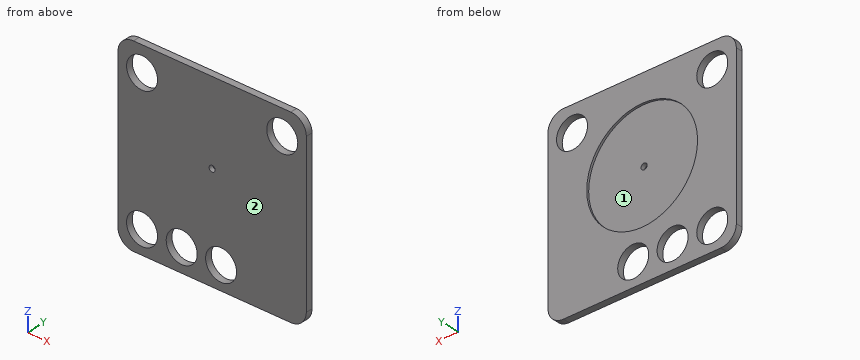
from build123d import *

# Parameters (mm, degrees)
SKETCH1_R           = 25
SKETCH1_R_2         = 7
BOSS_EXTRUDE1_DEPTH = 3
BOSS_EXTRUDE3_START = -2
SKETCH3_R           = 25
BOSS_EXTRUDE3_DEPTH = 2
SKETCH4_R           = 1.375
CUT_EXTRUDE1_DEPTH  = 2


with BuildPart() as part:
    # Sketch1 → Boss-Extrude1 (new body)
    with BuildSketch(Plane(origin=(0, 0, 0), x_dir=(1, 0, 0), z_dir=(0, 1, 0))):
        with BuildLine():
            Line((-32.846869633, -22.461451991), (38.153130367, -22.461451991))
            ThreePointArc((38.153130367, -22.461451991), (43.102877835, -20.411199459), (45.153130367, -15.461451991))
            Line((45.153130367, -15.461451991), (45.153130367, 55.538548009))
            ThreePointArc((45.153130367, 55.538548009), (43.102877835, 60.488295478), (38.153130367, 62.538548009))
            Line((38.153130367, 62.538548009), (-32.846869633, 62.538548009))
            ThreePointArc((-32.846869633, 62.538548009), (-37.796617101, 60.488295478), (-39.846869633, 55.538548009))
            Line((-39.846869633, 55.538548009), (-39.846869633, -15.461451991))
            ThreePointArc((-39.846869633, -15.461451991), (-37.796617101, -20.411199459), (-32.846869633, -22.461451991))
        make_face()
        with Locations(Location((2.653130367, 14.80701719, 0), (0, 0, 270))):
            Circle(SKETCH1_R, mode=Mode.SUBTRACT)
        with Locations(Location((-28.97725989, 52.02421358, 0), (0, 0, 270))):
            Circle(SKETCH1_R_2, mode=Mode.SUBTRACT)
        with Locations(Location((-11.083315318, 52.02421358, 0), (0, 0, 270))):
            Circle(SKETCH1_R_2, mode=Mode.SUBTRACT)
        with Locations(Location((6.69252819, 52.02421358, 0), (0, 0, 270))):
            Circle(SKETCH1_R_2, mode=Mode.SUBTRACT)
        with Locations(Location((-28.97725989, -11.117962427, 0), (0, 0, 270))):
            Circle(SKETCH1_R_2, mode=Mode.SUBTRACT)
        with Locations(Location((34.291639837, -11.117962427, 0), (0, 0, 270))):
            Circle(SKETCH1_R_2, mode=Mode.SUBTRACT)
    extrude(amount=-BOSS_EXTRUDE1_DEPTH)

    # Sketch3 → Boss-Extrude3 (add)
    with BuildSketch(Plane(origin=(0, -3, 0), x_dir=(-1, 0, 0), z_dir=(0, -1, 0)).offset(BOSS_EXTRUDE3_START)):
        with Locations(Location((-2.653130367, 14.80701719, 0), (0, 0, 270))):
            Circle(SKETCH3_R)
    extrude(amount=BOSS_EXTRUDE3_DEPTH)

    # Sketch4 → Cut-Extrude1 (cut)
    with BuildSketch(Plane(origin=(0, -1, 0), x_dir=(1, 0, 0), z_dir=(0, 1, 0))):
        with Locations(Location((2.653130367, 14.80701719, 0), (0, 0, 270))):
            Circle(SKETCH4_R)
    extrude(amount=-CUT_EXTRUDE1_DEPTH, mode=Mode.SUBTRACT)


solid = part.part
The model under review builds one solid part; all positions refer to its coordinate system, in mm. Face numbers are marked on the shaded views. Coordinates: 2 decimals unless noted, no trailing zeros. Loops run counter-clockwise (first coordinate to the right, second up) from the corner with the lowest first, then second, coordinate; pieces in that order, holes last. Notation, with made-up numbers: M 30.5,37 L 48.5,37 A15 cw 48.5,43 Z; hole C 45.25,-26.75 d10. An arc over 180 degrees is marked long. Put each result on its own line as item: value. Start each with the question number.
Q1. Add section D-D (z = -4). Write out the cut boundary in (x, y), and give its area (3 significant figures).
Q2. Wall thickness on line 1 (X direction, y = -1.75, z = -52.5); line 2 (Z direction, x = -28, y = -2.4); line 3 (X direction, y = -1.25, z = -51): over which ranges is each line inside the solid? List them lowest first.
Q3. Add section B-B (x = 26). Write out the cut boundary in (y, z), and give its area (3 significant figures).
Q4. Add section C-C (y = -1.75). Write out the cut boundary in (x, z) (3 decimals), and give its area (3 significant figures).
Q5. The part is to be moulded in two halves that separate along X. For the marked faces 1 and 2, say which applies: +X half, -X half, draft (parallel to the pull), parting line (faces both ways), or undercut.
Q6. Add section A-A (z = -46.5). Write out the cut boundary in (x, y).
Answers:
1. outline: M -39.85,-3 L 45.15,-3 L 45.15,0 L 25.2,0 L 25.2,-1 L -19.89,-1 L -19.89,0 L -39.85,0 Z
1. area: 210 mm^2
2. line 1: x = -39.85 to -35.96, -21.99 to -18.07, -4.1 to -0.29, 13.68 to 45.15
2. line 2: z = -62.54 to -58.96, -45.09 to 4.19, 18.05 to 22.46
2. line 3: x = -39.85 to -35.9, -22.05 to -18.01, -4.16 to -0.23, 13.62 to 45.15
3. outline: M -3,-62.54 L 0,-62.54 L 0,-23.75 L -1,-23.75 L -1,-5.87 L 0,-5.87 L 0,22.46 L -3,22.46 Z
3. area: 237 mm^2
4. outline: M -39.847,-55.539 A7 ccw -32.847,-62.539 L 38.153,-62.539 A7 ccw 45.153,-55.539 L 45.153,15.461 A7 ccw 38.153,22.461 L -32.847,22.461 A7 ccw -39.847,15.461 Z; hole C -28.977,-52.024 d14; hole C -28.977,11.118 d14; hole C -11.083,-52.024 d14; hole C 6.693,-52.024 d14; hole C 2.653,-14.807 d2.75; hole C 34.292,11.118 d14
4. area: 6,410 mm^2
5. face 1: undercut
5. face 2: draft
6. outline: M -39.85,-3 L -33.28,-3 L -33.28,0 L -39.85,0 Z; M -24.68,-3 L -15.38,-3 L -15.38,0 L -24.68,0 Z; M -6.78,-3 L 2.39,-3 L 2.39,0 L -6.78,0 Z; M 10.99,-3 L 45.15,-3 L 45.15,0 L 10.99,0 Z
